```python
from build123d import *

# Parameters (mm, degrees)
F0_R      = 9
F1_DEPTH  = 20
F2_R      = 0.75
F3_DEPTH  = 8
F4_R      = 9
F4_R_2    = 5.5
F5_DEPTH  = 30
F6_DEPTH  = 10
F7_R      = 3
F8_DEPTH  = 12.5
F10_D     = 3.2
F10_DEPTH = 7.25
F10_TIP   = 0.9613769904


with BuildPart() as f1:
    # F0 (on Front) → F1 (new body, symmetric)
    with BuildSketch(Plane.XZ):
        Circle(F0_R)
    extrude(amount=F1_DEPTH, both=True)

    # F2 (on face) → F3 (cut)
    with BuildSketch(Plane.XZ.offset(20)):
        with BuildLine():
            ThreePointArc((1, 7), (-0.0357371137, 7.9993612253), (-0.9974457174, 6.9285714286))
            ThreePointArc((-0.9974457174, 6.9285714286), (0, 6), (0.9974457174, 6.9285714286))
            ThreePointArc((0.9974457174, 6.9285714286), (0.9993612253, 6.9642628863), (1, 7))
        make_face()
        with Locations((0, 7)):
            Circle(F2_R, mode=Mode.SUBTRACT)
        with BuildLine():
            ThreePointArc((-5.0621778265, -3.5), (-5.5315479655, -2.6523963481), (-6.4990417278, -2.6004723841))
            ThreePointArc((-6.4990417278, -2.6004723841), (-6.9282032303, -4), (-5.5015960104, -4.3280990445))
            ThreePointArc((-5.5015960104, -4.3280990445), (-5.178837061, -3.9687313644), (-5.0621778265, -3.5))
        make_face()
        with Locations((-6.0621778265, -3.5)):
            Circle(F2_R, mode=Mode.SUBTRACT)
        with BuildLine():
            ThreePointArc((7.0621778265, -3.5), (6.9097814784, -2.969370139), (6.4990417278, -2.6004723841))
            ThreePointArc((6.4990417278, -2.6004723841), (5.1961524227, -3), (5.5015960104, -4.3280990445))
            ThreePointArc((5.5015960104, -4.3280990445), (6.5309091909, -4.3833407655), (7.0621778265, -3.5))
        make_face()
        with Locations((6.0621778265, -3.5)):
            Circle(F2_R, mode=Mode.SUBTRACT)
    extrude(amount=-F3_DEPTH, mode=Mode.SUBTRACT)

    # F4 (on face) → F5 (cut)
    with BuildSketch(Plane(origin=(0, 20, 0), x_dir=(-1, 0, 0), z_dir=(0, 1, 0))):
        Circle(F4_R)
        Circle(F4_R_2, mode=Mode.SUBTRACT)
    extrude(amount=-F5_DEPTH, mode=Mode.SUBTRACT)

    # F2 (on face) → F6 (cut)
    with BuildSketch(Plane.XZ.offset(20)):
        with Locations((-6.0621778265, -3.5)):
            Circle(F2_R)
        with Locations((0, 7)):
            Circle(F2_R)
        with Locations((6.0621778265, -3.5)):
            Circle(F2_R)
    extrude(amount=-F6_DEPTH, mode=Mode.SUBTRACT)

    # F7 (on Top) → F8 (cut, symmetric)
    with BuildSketch(Plane.XY):
        with Locations((0, 12)):
            Circle(F7_R)
    extrude(amount=F8_DEPTH, both=True, mode=Mode.SUBTRACT)

    # F10
    with Locations(Plane(origin=(0, 20, 0), x_dir=(-1, 0, 0), z_dir=(0, 1, 0))):
        with Locations((0, 0)):
            Hole(F10_D / 2, depth=F10_DEPTH)
            with Locations((0, 0, -(F10_DEPTH + F10_TIP / 2))):  # 118° drill point
                Cone(0, F10_D / 2, F10_TIP, mode=Mode.SUBTRACT)


solid = f1.part
```
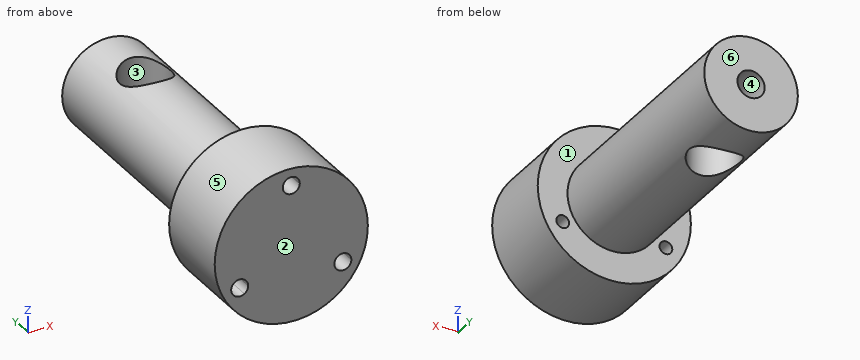
Geometry check sheet. Reference: the model listing, model coordinates, mm. Face numbers are marked on the shaded views. A direction names the side the tool comes from. Coordinates: 2 decimals unless noted, no trailing zeros. Write each loop counter-clockwise with the first axis right and the second up, starting at its lowest first coordinate (ties: lowest second). Pieces come first, ordered by that corner, then holes. Notation, with made-up numbers: M -1,60.25 L 6,60.25 A10 ccw 6,70.25 Z; hole C -26,23 d3. An arc over 180 degrees is marked long. One line per item, written item: value. Start each with the question number.
(1) Sectioned sample at B-B, the plane z = 5. Enter the section's corners in (x, y).
(2) Sectioned sample at C-C, the plane y = -16. Enter the section's corners in (x, z).
(3) Sectioned sample at A-A, the plane x = 0. Enter the section's corners in (y, z), and give its area (3 significant figures).
(4) Depth check by flat-ended pin: pin 1 (6 mm diameter, centred on x = -4.5, y = 9, fed in from +Z); pin 2 (3 mm diameter, centred on y = -0.5, z = -3, fed in from -X); pin 3 (1.7 mm diameter, centred on x = 0, z = 7, fed in from -Y); pin 4 (1.2 mm diameter, centred on x = -6.06, z = -3.5, fed in from +Y). Enter the tip coordinate at first touch or a pass-through.
(5) Scan lines: line 1 along Z through (x, y) = (0, 18.35); line 2 along Z through (x, y) = (0, -11.3); line 3 along Y through (x, z) = (-4.25, 5). Record each from-to range of solid material in increasing order. Write a range as [from, to].
(6) Release check for a two-part mould opening along X. For the marked faces 3, 4, 5 and 6 record: released by +X, released by -X, zero draft, split by the parting line, or undercut.
(7) Tool access check on the marked faces 1 and 2. Record the directions out of +Z, -Z, +X, -X, +Y, -Y that give a thin tool (end or side, any length) a straight path to the whole face; none if there is none.
(8) Sectioned sample at D-D, the plane y = 16. Enter the section's corners in (x, z), and give its area (3 significant figures).
Filled sheet:
1. outline: M -7.48,-20 L 7.48,-20 L 7.48,-10 L 2.29,-10 L 2.29,10.06 A3 cw -2.29,10.06 L -2.29,-10 L -7.48,-10 Z; M -2.29,13.94 A3 cw 2.29,13.94 L 2.29,20 L -2.29,20 Z
2. outline: C 0,0 d18; hole C -6.06,-3.5 d2; hole C 0,7 d2; hole C 6.06,-3.5 d2
3. outline: M -20,-9 L -10,-9 L -10,-5.5 L 9,-5.5 L 9,5.5 L -10,5.5 L -10,6.25 L -12,6.25 L -12,6 L -20,6 Z; M -20,8 L -12,8 L -12,7.75 L -10,7.75 L -10,9 L -20,9 Z; M 15,-5.5 L 20,-5.5 L 20,-1.6 L 15,-1.6 Z; M 15,1.6 L 20,1.6 L 20,5.5 L 15,5.5 Z
3. area: 409 mm²
4. pin 1: z = 5.29
4. pin 2: x = -5.29
4. pin 3: y = -12
4. pin 4: through
5. line 1: [-5.5, -1.6], [1.6, 5.5]
5. line 2: [-9, 6.25], [7.75, 9]
5. line 3: [-20, -10]
6. face 3: undercut
6. face 4: undercut
6. face 5: split by the parting line
6. face 6: zero draft
7. face 1: +Y
7. face 2: +Z, -Z, +X, -X, -Y
8. outline: C 0,0 d11; hole C 0,0 d3.2
8. area: 87.0 mm²
